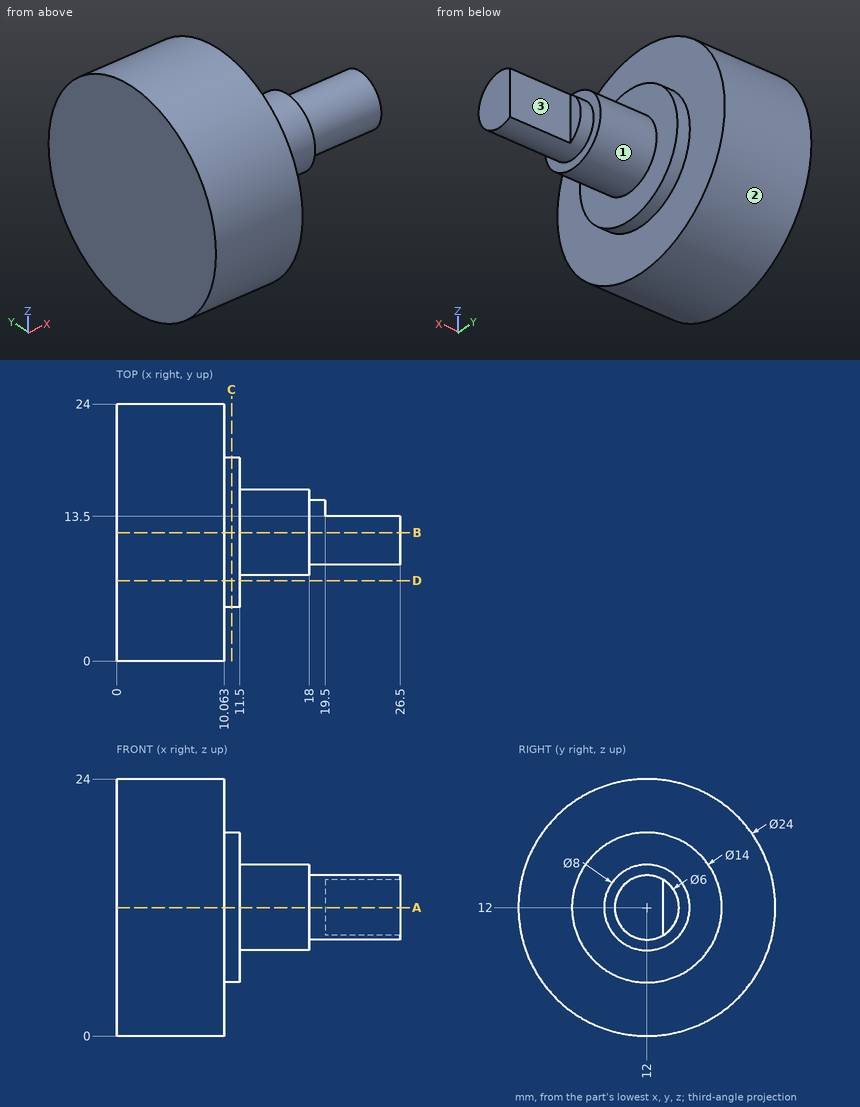
Source: three-view drawing plus pictorial views. Frame: mm from the lowest corner of the part. A direction names the side the tool comes from. Give positions to 0.01 mm unless a question says otherwise; leave off trailing zeros. Order: outer loops, then holes, each group sorted by start corner. A loop starts at its lowest first (then second) coordinate and runs counter-clockwise, first axis right, second up. Notation, with made-up numbers: (51, -2) - (105, -2) arc R16 cw to (105, 6) - close; hole circle Ø4 at (24, -15). An arc over 180 degrees is marked (long way). Answer as a JSON object with one key per item and string values. Group by question number.
Q1. Cut plane B-B, the plane y = 12. Output: boundary loops of the cut face in (x, z).
Q2. First-contact query: pin 1 Ø3 at (x, z) = (8, 5.5) entering from +Y; pin 2 Ø4 at (x, z) = (24, 12) entering from +Y; pin 3 Ø8 at (x, y) = (8.5, 5) entering from -Z. Flat tips, straight axial feed; report the tip coordinate or a pass-through.
Q3. Set-up query: the marked faces 1, 2 and 3. Return all of +Z, -Z, +X, -X, +Y, -Y with unobstructed straight access to the full face (end or side cutting, diameter ignored); none if empty.
Q4. Cut plane A-A, the plane z = 12. Output: boundary loops of the cut face in (x, y), then the cut area to 3 significant figures.
Q5. Line query: probe 1 along Z at (x, y) = (20, 10.5); probe 2 along X at (y, z) = (18.25, 15.5); probe 3 along X at (y, z) = (8.25, 6.25). Output: solid intervals per line, ascending.
Q6. Cut plane C-C, the plane x = 10.75. Output: boundary loops of the cut face in (y, z), then the cut area to 3 significant figures.
Q7. Cut plane D-D, the plane y = 7.5. Output: boundary loops of the cut face in (x, z), then the cut area to 3 significant figures.
Results:
{
 "1": {"outline": "(0, 0) - (10.06, 0) - (10.06, 5) - (11.5, 5) - (11.5, 8) - (18, 8) - (18, 9) - (26.5, 9) - (26.5, 15) - (18, 15) - (18, 16) - (11.5, 16) - (11.5, 19) - (10.06, 19) - (10.06, 24) - (0, 24) - close"},
 "2": {"pin 1": "y = 22.91", "pin 2": "y = 13.5", "pin 3": "z = 0.38"},
 "3": {"face 1": "+X", "face 2": "+X, -X", "face 3": "+Z, -Z, +X, +Y"},
 "4": {"outline": "(0, 0) - (10.06, 0) - (10.06, 5) - (11.5, 5) - (11.5, 8) - (18, 8) - (18, 9) - (26.5, 9) - (26.5, 13.5) - (19.5, 13.5) - (19.5, 15) - (18, 15) - (18, 16) - (11.5, 16) - (11.5, 19) - (10.06, 19) - (10.06, 24) - (0, 24) - close", "area": "354 mm^2"},
 "5": {"probe 1": "9.4 to 14.6", "probe 2": "0 to 10.06", "probe 3": "0 to 11.5"},
 "6": {"outline": "circle Ø14 at (12, 12)", "area": "154 mm^2"},
 "7": {"outline": "(0, 0.88) - (10.06, 0.88) - (10.06, 6.64) - (11.5, 6.64) - (11.5, 17.36) - (10.06, 17.36) - (10.06, 23.12) - (0, 23.12) - close", "area": "239 mm^2"}
}
